from build123d import *

# Parameters (mm, degrees)
CHAMFER1_SIZE  = 1.27
CHAMFER1_SIZE2 = 0.340295474
FILLET1_R      = 0.254


with BuildPart() as part:
    # Sketch1 → Revolve1 (revolve)
    with BuildSketch(Plane(origin=(0, 0, 0), x_dir=(0, 0, -1), z_dir=(1, 0, 0))):
        Polygon((0, 5.08), (0, 13.462), (2.794, 13.462), (2.794, 11.43), (6.35, 11.43), (6.35, 13.462), (10.16, 13.462), (10.16, 12.065), (17.78, 12.065), (17.78, 6.731), (5.08, 6.731), (5.08, 0), (0, 0), (-5.08, 0), (-5.08, 5.08), align=None)
    revolve(axis=Axis((0, 0, -5.08), (0, 0, 1)))

    # Chamfer1
    chamfer1_edges = [part.edges().sort_by_distance(p)[0] for p in [
        (0, -12.065, -17.78),
    ]]
    chamfer1_side = [part.faces().sort_by_distance(p)[0] for p in [
        (0, -12.065, -13.97),
    ]]
    chamfer(chamfer1_edges, length=CHAMFER1_SIZE, length2=CHAMFER1_SIZE2, reference=chamfer1_side[0])

    # Fillet1
    fillet1_edges = [part.edges().sort_by_distance(p)[0] for p in [
        (0, -13.462, -6.35),
        (0, -11.43, -6.35),
        (0, -11.43, -2.794),
        (0, -13.462, -2.794),
    ]]
    fillet(fillet1_edges, radius=FILLET1_R)


solid = part.part
Source: CAD feature listing. Evaluate the final solid. Frame: model axes, mm. A direction names the side the tool comes from. Give positions to 0.01 mm unless a question says otherwise; leave off trailing zeros. Write each loop counter-clockwise with the first axis right and the second up, starting at its lowest first coordinate (ties: lowest second). Pieces come first, ordered by that corner, then holes. Notation, with made-up numbers: (-33, 34) -> (-16, 34) arc R21 cw to (-16, 56) -> close; hole circle Ø1 at (30, 33.5). An arc over 180 degrees is marked (long way). Return JSON: item names as keys, results as strings. Group by question number.
1. Access query for faces 1 (the face through (0, -6, 0)), 2 (the face through (8.191, -10.683, -1.288)), 3 (the face through (4.1, -5.34, -11.34)), 4 (the face through (12, 1, -2.794)). Directions: +Z, -Z, +X, -X, +Y, -Y. A direction counts if a zero-diameter tool reaches every point of the face in a straight line with its end or side. Return the directions, or none.
2. Pin query (flat end, axial travel): pin 1 Ø1 at (x, z) = (-10.5, -12.5) entering from -Y; pin 2 Ø6 at (x, y) = (4.5, 11) entering from -Z; pin 3 Ø1.5 at (x, z) = (-4, -5) entering from -Y; pin 4 Ø5 at (x, z) = (-8, -8.5) entering from -Y. Return the tip coordinate at first contact, or that it passes through.
3. Mould query, pull axis Z, two halves, no side actions, for faces 5 (the face through (0, 0, -5.08)), 6 (the face through (12, -1, -6.35)), 7 (the face through (-3.433, 10.902, -4.593)), 8 (the face through (-5.037, -0.661, 2.504)). Classes: +Z half, -Z half, draft (parallel to the pull), parting line (faces both ways), or undercut.
4. Section D-D, the plane z = -0.75. Output: boundary loops of the cut face in (x, y), then the cut area to 3 significant figures.
5. Material intervals for line 1 (Y direction, x = 0, z = -15) (3 decimals); line 2 (Z direction, x = 6, y = -10), sorted ascending. Write a range as from..to.
6. Section A-A, the plane z = -12. Output: boundary loops of the cut face in (x, y) (3 decimals), then the cut area to 3 significant figures.
Determined:
{
 "1": {"face 1": "+Z", "face 2": "+Z, -Z", "face 3": "-Z", "face 4": "none"},
 "2": {"pin 1": "stops at y = -6.75", "pin 2": "stops at z = -17.78", "pin 3": "stops at y = -10.96", "pin 4": "stops at y = -12.29"},
 "3": {"face 5": "-Z half", "face 6": "undercut", "face 7": "undercut", "face 8": "draft"},
 "4": {"outline": "circle Ø26.92 at (0, 0)", "area": "569 mm2"},
 "5": {"line 1": "y = -12.065..-6.731, 6.731..12.065", "line 2": "z = -17.78..-6.35, -2.79..0"},
 "6": {"outline": "circle Ø24.13 at (0, 0); hole circle Ø13.462 at (0, 0)", "area": "315 mm2"}
}
